For this review, take the finished solid that the model builds, in its own axes (mm). A direction names the side the tool comes from. Give positions to 0.01 mm unless a question says otherwise; leave off trailing zeros. Loops run counter-clockwise (first coordinate to the right, second up) from the corner with the lowest first, then second, coordinate; pieces in that order, holes last. Notation, with made-up numbers: (-13.5, 46) - (-8.5, 46) arc R12 cw to (-8.5, 52) - close; hole circle Ø7 at (-27, 81.5). An arc over 180 degrees is marked (long way). Use CSV: the item, a comma, the result in double quotes. Start each with the question number.
1. Take a section at A-A on x = -19.5. Give the boundary of the cut face in (y, z).
2. Wall thickness on line 1 (Y direction, x = 10.5, z = 2.25); line 2 (Y direction, x = 10.5, z = 6); line 3 (Y direction, x = -74, z = 5.5): over which ranges is each line inside the solid? List them lowest first.
3. For pin 1 (8 mm diameter, centred on y = 9, z = 15, fed in from -X); pin 2 (12 mm diameter, centred on x = -73.5, y = -10, fed in from -Z); pin 3 (3 mm diameter, centred on y = -0.5, z = 28.5, fed in from -X); pin 4 (10 mm diameter, centred on x = -91.5, z = 7.5, fed in from -Y), all flat-tipped, find the tip position at first contact; note any pin that passes through.
4. Mouldability with a two-part tool opening along Z and no side actions: class faces 5 (the cylindrical face through (-85, -2, 42.6)), 6 (the flat face through (-20, 0, 5)), 7 (the flat face through (-24, 0, 0)) as pulls with the +Z half, pulls with the -Z half, needs draft (parallel to the pull), parting line crosses it, or undercut.
5. For faces 1 (the flat face through (12.5, 0, 2)), 2 (the flat face through (12, -3, 8)), 3 (the flat face through (-94.176, -1.772, 42.575)), 4 (the cylindrical face through (12.21, 10.07, 6.48)), list the 3-axis set-ups (+Z, -Z, +X, -X, +Y, -Y) from which the entire face can be reached by the end or side of a thin tool; tool diameter is ignored.
6. Take a section at B-B on z = 44.5. State how many separate pieces and enclosed holes the cut face has, plus the area to 3 significant figures.
Autodesk Fusion 360 part; units mm, degrees
sketch "Sketch1" plane through (0, 0, 0) normal (0, 0, 1) x (1, 0, 0)
  circle A0 centre (10.5, -3.138) radius 1.2
  line L0 (-10.5, 12.5) -> (10.5, 12.5)
  arc A1 (-12.5, -10.5) -> (-10.5, -12.5) centre (-10.5, -10.5) ccw
  circle A2 centre (-10.5, -3.138) radius 1.2
  arc A3 (10.5, -12.5) -> (12.5, -10.5) centre (10.5, -10.5) ccw
  circle A4 centre (-10.5, 9.362) radius 1.2
  arc A5 (-10.5, 12.5) -> (-12.5, 10.5) centre (-10.5, 10.5) ccw
  line L1 (-12.5, -10.5) -> (-12.5, 10.5)
  line L2 (12.5, 10.5) -> (12.5, -10.5)
  arc A6 (12.5, 10.5) -> (10.5, 12.5) centre (10.5, 10.5) ccw
  circle A7 centre (10.5, 9.362) radius 1.2
  line L3 (10.5, -12.5) -> (-10.5, -12.5)
  point P0 (-12.5, 12.5)
  point P1 (12.5, 12.5)
  point P2 (-12.5, -12.5)
  dimension "d1" = 25
  dimension "d2" = 25
  dimension "d3" = 2.4
  dimension "d4" = 2
  dimension "d5" = 2
  dimension "d6" = 2
  dimension "d7" = 2
  dimension "d8" = 2
  dimension "d9" = 2
  dimension "d10" = 2
  dimension "d11" = 12.5
  dimension "d12" = 12.5
  dimension "d13" = 21.862
  dimension "d14" = 21.862
  dimension "d15" = 9.362
  dimension "d16" = 9.362
  dimension "d17" = 12.5
  dimension "d18" = 12.5
extrude "Extrude1" add sketch "Sketch1" along normal blind 5
sketch "Sketch2" plane through (0, 0, 5) normal (0, 0, 1) x (1, 0, 0)
  circle A0 centre (-10.5, 9.362) radius 1.2
  circle A1 centre (10.5, -3.138) radius 1.2
  circle A2 centre (-10.5, -3.138) radius 1.2
  circle A3 centre (10.5, 9.362) radius 1.2
  arc A4 (12.5, 10.5) -> (10.5, 12.5) centre (10.5, 10.5) ccw
  line L0 (10.5, 12.5) -> (-10.5, 12.5)
  arc A5 (-10.5, 12.5) -> (-12.5, 10.5) centre (-10.5, 10.5) ccw
  line L1 (-12.5, 10.5) -> (-12.5, -10.5)
  arc A6 (-12.5, -10.5) -> (-10.5, -12.5) centre (-10.5, -10.5) ccw
  line L2 (-10.5, -12.5) -> (10.5, -12.5)
  arc A7 (10.5, -12.5) -> (12.5, -10.5) centre (10.5, -10.5) ccw
  line L3 (12.5, -10.5) -> (12.5, 10.5)
  circle A8 centre (-10.5, 9.362) radius 1.85
  circle A9 centre (10.5, 9.362) radius 1.85
  circle A10 centre (10.5, -3.138) radius 1.85
  circle A11 centre (-10.5, -3.138) radius 1.85
  dimension "d21" = 3.7
  dimension "d22" = 3.7
  dimension "d23" = 3.7
  dimension "d24" = 3.7
extrude "Extrude2" add sketch "Sketch2" along normal blind 3 contours A8 | A9 | A10 | A11
sketch "Sketch3" plane through (-12.5, 0, 0) normal (-1, 0, 0) x (0, 0, 1)
  line L0 (0, 10.5) -> (0, -10.5)
  line L1 (0, -10.5) -> (5, -10.5)
  line L2 (5, -10.5) -> (5, 10.5)
  line L3 (5, 10.5) -> (0, 10.5)
  line L4 (0, 7.5) -> (5, 7.5)
  line L5 (5, 7.5) -> (5, -7.5)
  line L6 (5, -7.5) -> (0, -7.5)
  line L7 (0, -7.5) -> (0, 7.5)
  dimension "d29" = 3
  dimension "d30" = 3
extrude "Extrude3" add sketch "Sketch3" along normal blind 68 contours L0 L2 L4 L5 L6 L7
fillet "Fillet1" radius 3 2 edges at (-12.5, 7.5, 2.5) (-12.5, -7.5, 2.5)
sketch "Sketch5" plane through (0, 7.5, 0) normal (0, 1, 0) x (-1, 0, 0)
  line L0 (15.5, 5) -> (15.5, 0)
  line L1 (15.5, 0) -> (80.5, 0)
  line L2 (80.5, 0) -> (80.5, 5)
  line L3 (80.5, 5) -> (15.5, 5)
  line L4 (80.5, 0) -> (94.2374, 0)
  line L5 (94.2374, 0) -> (80.5, 5)
  line L6 (84.001, 0) -> (85.1985, 3.2899)
  dimension "d38" = 20
  dimension "d39" = 5
  dimension "d40" = 5
extrude "Extrude5" add sketch "Sketch5" against normal up to surface (15 mm away) contours L2 L4 L5 L6
sketch "Sketch6" plane through (-11.0237, 0, 30.2873) normal (-0.342, 0, 0.9397) x (0.9397, 0, 0.342)
  line L0 (-78.9352, -7.5) -> (-73.9352, -7.5)
  line L1 (-73.9352, -7.5) -> (-73.9352, 7.5)
  line L2 (-73.9352, 7.5) -> (-78.9352, 7.5)
  line L3 (-78.9352, 7.5) -> (-78.9352, -7.5)
  line L4 (-78.9352, 7.5) -> (-73.9352, 7.5)
  line L5 (-73.9352, 7.5) -> (-73.9352, -7.5)
  line L6 (-73.9352, -7.5) -> (-78.9352, -7.5)
  line L7 (-78.9352, -7.5) -> (-78.9352, 7.5)
extrude "Extrude6" add sketch "Sketch6" along normal blind 55.398
sketch "Sketch7" plane through (-69.4763, 0, -25.2873) normal (0.9397, 0, 0.342) x (0.342, 0, -0.9397)
  line L0 (-32.2311, -7.5) -> (-32.2311, 7.5)
  line L1 (-32.2311, 7.5) -> (-87.6291, 7.5)
  line L2 (-87.6291, 7.5) -> (-87.6291, -7.5)
  line L3 (-87.6291, -7.5) -> (-32.2311, -7.5)
  line L4 (-87.6291, 0) -> (-32.2311, 0) construction
  circle A0 centre (-80.1291, 0) radius 2.25
  circle A1 centre (-70.1291, 0) radius 2.25
  dimension "d45" = 4.5
  dimension "d46" = 4.5
  dimension "d47" = 7.5
  dimension "d48" = 10
extrude "Extrude7" cut sketch "Sketch7" against normal up to surface (5 mm away) contours A0 | A1
sketch "Sketch8" plane through (0, 7.5, 0) normal (0, 1, 0) x (-1, 0, 0)
  line L0 (15.5, 5) -> (15.5, 0)
  line L1 (15.5, 0) -> (84.001, 0)
  line L2 (84.001, 0) -> (104.1457, 55.347)
  line L3 (104.1457, 55.347) -> (99.4472, 57.0571)
  line L4 (99.4472, 57.0571) -> (80.5, 5)
  line L5 (80.5, 5) -> (15.5, 5)
  line L6 (74.0085, 5) -> (93.7151, 59.1434)
  line L7 (93.7151, 59.1434) -> (89.0166, 60.8535)
  line L8 (89.0166, 60.8535) -> (68.6876, 5)
  line L9 (99.4472, 57.0571) -> (93.7151, 59.1434) construction
  dimension "d51" = 6.1
  dimension "d52" = 5
extrude "Extrude8" add sketch "Sketch8" against normal up to surface (15 mm away) contours L5 L6 L7 L8
sketch "Sketch9" plane through (-59.0457, 0, -21.4909) normal (0.9397, 0, 0.342) x (0.342, 0, -0.9397)
  line L0 (-87.6291, -7.5) -> (-28.191, -7.5)
  line L1 (-28.191, -7.5) -> (-28.191, 7.5)
  line L2 (-28.191, 7.5) -> (-87.6291, 7.5)
  line L3 (-87.6291, 7.5) -> (-87.6291, -7.5)
  circle A0 centre (-80.1291, 0) radius 2.25
  circle A1 centre (-70.1291, 0) radius 2.25
extrude "Extrude9" cut sketch "Sketch9" against normal up to surface (5 mm away) contours A0 | A1
sketch "Sketch10" plane through (0, 7.5, 0) normal (0, 1, 0) x (-1, 0, 0)
  line L0 (15.5, 5) -> (15.5, 0)
  line L1 (15.5, 0) -> (84.001, 0)
  line L2 (84.001, 0) -> (104.1457, 55.347)
  line L3 (104.1457, 55.347) -> (99.4472, 57.0571)
  line L4 (99.4472, 57.0571) -> (80.5, 5)
  line L5 (80.5, 5) -> (74.0085, 5)
  line L6 (74.0085, 5) -> (93.7151, 59.1434)
  line L7 (93.7151, 59.1434) -> (89.0166, 60.8535)
  line L8 (89.0166, 60.8535) -> (68.6876, 5)
  line L9 (68.6876, 5) -> (15.5, 5)
  line L10 (89.0505, 28.4923) -> (83.3184, 30.5786)
  dimension "d57" = 30.398
extrude "Extrude10" add sketch "Sketch10" against normal up to surface (15 mm away) contours L4 L5 L6 L10
equation "d17 = d11"
equation "d18 = d12"
equation "d22 = d21"
equation "d23 = d21"
equation "d24 = d21"
equation "d30 = d29"
equation "d40 = d39"
equation "d43 = 19.898 mm + 7.5 mm + 28 mm"
equation "d46 = d45"
equation "d57 = d43 - 25 mm"
Check result:
1,outline,"(-7.5, 0) - (7.5, 0) - (7.5, 5) - (-7.5, 5) - close"
2,line 1,"y = -12.5 to -4.34, -1.94 to 8.16, 10.56 to 12.5"
2,line 2,"y = -4.99 to -4.34, -1.94 to -1.29, 7.51 to 8.16, 10.56 to 11.21"
2,line 3,"y = -7.5 to 7.5"
3,pin 1,"stops at x = -90.81"
3,pin 2,"stops at z = 0"
3,pin 3,"stops at x = -94.92"
3,pin 4,"stops at y = -7.5"
4,face 5,"undercut"
4,face 6,"pulls with the +Z half"
4,face 7,"pulls with the -Z half"
5,face 1,"+Z, -Z, +X, +Y, -Y"
5,face 2,"+Z, +X, +Y, -Y"
5,face 3,"+Y, -Y"
5,face 4,"+Z"
6,separate pieces,"3"
6,enclosed holes,"0"
6,area,"139 mm²"
